from build123d import *

# Parameters (mm, degrees)
F0_W     = 762
F0_H     = 1778
F1_DEPTH = 1193.8
F3_DEPTH = 1524
F4_W     = 25.4
F4_H     = 419.191256
F4_W_2   = 25.17225
F5_DEPTH = 127


with BuildPart() as f1:
    # F0 (on Front) → F1 (new body)
    with BuildSketch(Plane.XZ):
        Rectangle(F0_W, F0_H)
    extrude(amount=F1_DEPTH)

    # F2 (on face) → F3 (cut)
    with BuildSketch(Plane(origin=(0, 0, 0), x_dir=(-1, 0, 0), z_dir=(0, 1, 0))):
        Polygon((381, 889), (279.4, 889), (381, 430.121779), align=None)
    extrude(amount=-F3_DEPTH, mode=Mode.SUBTRACT)

    # F4 (on face) → F5 (cut)
    with BuildSketch(Plane(origin=(-453.978061, 0, 100.515058), x_dir=(0, -1, 0), z_dir=(-0.976355, 0, 0.216174))):
        with Locations((88.9, 572.58471)):
            Rectangle(F4_W, F4_H)
        with Locations((139.7, 572.58471)):
            Rectangle(F4_W, F4_H)
        with Locations((190.5, 572.58471)):
            Rectangle(F4_W, F4_H)
        with Locations((241.3, 572.58471)):
            Rectangle(F4_W, F4_H)
        with Locations((292.1, 572.58471)):
            Rectangle(F4_W, F4_H)
        with Locations((342.9, 572.58471)):
            Rectangle(F4_W, F4_H)
        with Locations((393.7, 572.58471)):
            Rectangle(F4_W, F4_H)
        with Locations((444.5, 572.58471)):
            Rectangle(F4_W, F4_H)
        with Locations((495.3, 572.58471)):
            Rectangle(F4_W, F4_H)
        with Locations((546.1, 572.58471)):
            Rectangle(F4_W, F4_H)
        with Locations((596.9, 572.58471)):
            Rectangle(F4_W, F4_H)
        with Locations((647.7, 572.58471)):
            Rectangle(F4_W, F4_H)
        with Locations((698.386125, 572.58471)):
            Rectangle(F4_W_2, F4_H)
        with Locations((749.07225, 572.58471)):
            Rectangle(F4_W, F4_H)
        with Locations((799.87225, 572.58471)):
            Rectangle(F4_W, F4_H)
        with Locations((850.67225, 572.58471)):
            Rectangle(F4_W, F4_H)
        with Locations((901.47225, 572.58471)):
            Rectangle(F4_W, F4_H)
        with Locations((952.27225, 572.58471)):
            Rectangle(F4_W, F4_H)
        with Locations((1017.819324, 572.58471)):
            Rectangle(F4_W, F4_H)
        with Locations((1068.619324, 572.58471)):
            Rectangle(F4_W, F4_H)
    extrude(amount=-F5_DEPTH, mode=Mode.SUBTRACT)


solid = f1.part
Can you work these out from the model? Positions are in its coordinate system, mm. Give positions to 0.01 mm unless a question says otherwise; leave off trailing zeros. Answer as a JSON object with one key per item and string values.
Q1. If I drill on L1, parallel to Z at x = -254.5, y = -101; L2, parallel to Z at x = -260.5, y = -789; L3, parallel to X at y = -844.5, z = 760, over which ranges is the centre line in solid material (lowest first)?
Geometry says:
{"L1": "-889 to 428.13, 857.47 to 889", "L2": "-889 to 429.46, 858.8 to 889", "L3": "-177.89 to 381"}
Q2. Imagine slicing it at A-A on x = -211.5. Give the number of separate pieces and of enclosed holes in the cut face, plus the area to 3 significant figures.
Geometry says:
{"separate pieces": "1", "enclosed holes": "20", "area": "2,000,000 mm²"}
Q3. If we mould it in two halves opening along Z, with no side actions, what happens to faces 1 (the flat face through (-270, -254, 643)), 2 (the flat face through (-205.57, -545.92, 634.97)), 3 (the flat face through (46, -589, 889)), 4 (the flat face through (381, -589, -12))? For each: pulls with the +Z half, pulls with the -Z half, needs draft (parallel to the pull), parting line crosses it, or undercut.
Geometry says:
{"face 1": "undercut", "face 2": "undercut", "face 3": "pulls with the +Z half", "face 4": "needs draft"}
